from build123d import *

# Parameters (mm, degrees)
SKETCH_1_R                        = 1.6
SM_BASE_FLANGE_1_DEPTH            = 1
SKETCH_2_R                        = 3
EXTRUDE_1_DEPTH                   = 2
HOLE_WIZARD_M3_1_D                = 2.5
SM_EDGE_FLANGE_1_STRIP_W          = 6
SM_EDGE_FLANGE_1_STRIP_H          = 1
SM_EDGE_FLANGE_1_STRIP_CUT_DEPTH  = 177.34
SM_EDGE_FLANGE_1_RELIEF_W         = 8
SM_EDGE_FLANGE_1_RELIEF_H         = 2
SM_EDGE_FLANGE_1_RELIEF_CUT_DEPTH = 1
SM_EDGE_FLANGE_1_DEPTH            = 177.34
SM_EDGE_FLANGE_1_FLAT_DEPTH       = 1
SKETCH_8_R                        = 3
EXTRUDE_2_DEPTH                   = 2
HOLE_WIZARD_M3_2_D                = 2.5


# Sheet-metal steps are written as plain solids
with BuildPart() as part:
    # Sketch 1 → 基体-法兰1 (new body)
    with BuildSketch(Plane(origin=(0, 0, 0), x_dir=(1, 0, 0), z_dir=(0, 1, 0))):
        with BuildLine():
            Line((-113.67, 31.388001247), (-113.67, -28.611998753))
            ThreePointArc((-113.67, -28.611998753), (-112.791320344, -30.733319096), (-110.67, -31.611998753))
            Line((-110.67, -31.611998753), (110.67, -31.611998753))
            ThreePointArc((110.67, -31.611998753), (112.791320344, -30.733319096), (113.67, -28.611998753))
            Line((113.67, -28.611998753), (113.67, -8.25463944))
            ThreePointArc((113.67, -8.25463944), (113.441638598, -7.106589143), (112.791320344, -6.133319096))
            Line((112.791320344, -6.133319096), (55.148679656, 51.509321591))
            ThreePointArc((55.148679656, 51.509321591), (54.17540961, 52.159639845), (53.027359313, 52.388001247))
            Line((53.027359313, 52.388001247), (-2.67, 52.388001247))
            ThreePointArc((-2.67, 52.388001247), (-4.084213562, 51.80221481), (-4.67, 50.388001247))
            Line((-4.67, 50.388001247), (-4.67, 33.388001247))
            Line((-4.67, 33.388001247), (-111.67, 33.388001247))
            ThreePointArc((-111.67, 33.388001247), (-113.084213562, 32.80221481), (-113.67, 31.388001247))
        make_face()
        with Locations(Location((-105.67, -13.611998753, 0), (0, 0, 270))):
            Circle(SKETCH_1_R, mode=Mode.SUBTRACT)
        with Locations(Location((-105.67, 13.388001247, 0), (0, 0, 270))):
            Circle(SKETCH_1_R, mode=Mode.SUBTRACT)
        with Locations(Location((-89.67, 25.388001247, 0), (0, 0, 270))):
            Circle(SKETCH_1_R, mode=Mode.SUBTRACT)
        with Locations(Location((-25.67, 25.388001247, 0), (0, 0, 270))):
            Circle(SKETCH_1_R, mode=Mode.SUBTRACT)
        with Locations(Location((22.33, 44.388001247, 0), (0, 0, 270))):
            Circle(SKETCH_1_R, mode=Mode.SUBTRACT)
        with Locations(Location((60.516291501, 34.828001247, 0), (0, 0, 270))):
            Circle(SKETCH_1_R, mode=Mode.SUBTRACT)
        with Locations(Location((96.116291501, -0.771998753, 0), (0, 0, 270))):
            Circle(SKETCH_1_R, mode=Mode.SUBTRACT)
        with Locations(Location((105.67, -19.111998753, 0), (0, 0, 270))):
            Circle(SKETCH_1_R, mode=Mode.SUBTRACT)
        with BuildLine():
            Line((-43.83, 11.388001247), (5.17, 11.388001247))
            ThreePointArc((5.17, 11.388001247), (5.523553391, 11.241554638), (5.67, 10.888001247))
            Line((5.67, 10.888001247), (5.67, -16.111998753))
            ThreePointArc((5.67, -16.111998753), (5.523553391, -16.465552143), (5.17, -16.611998753))
            Line((5.17, -16.611998753), (-43.83, -16.611998753))
            ThreePointArc((-43.83, -16.611998753), (-44.183553391, -16.465552143), (-44.33, -16.111998753))
            Line((-44.33, -16.111998753), (-44.33, 10.888001247))
            ThreePointArc((-44.33, 10.888001247), (-44.183553391, 11.241554638), (-43.83, 11.388001247))
        make_face(mode=Mode.SUBTRACT)
    extrude(amount=-SM_BASE_FLANGE_1_DEPTH)

    # Sketch 2 → 凸台-拉伸1 (add)
    with BuildSketch(Plane.XZ.offset(1)):
        with Locations(Location((-19.33, -17.388001247, 0), (0, 0, 90))):
            Circle(SKETCH_2_R)
        with Locations(Location((-19.33, 22.611998753, 0), (0, 0, 90))):
            Circle(SKETCH_2_R)
    extrude(amount=EXTRUDE_1_DEPTH)

    # M3 螺纹孔1 (through all)
    with Locations(Plane(origin=(0, -3, 0), x_dir=(-1, 0, 0), z_dir=(0, -1, 0))):
        with Locations((19.33, 17.388001247), (19.33, -22.611998753)):
            Hole(HOLE_WIZARD_M3_1_D / 2)

    # 边线-法兰1 strip (across the edge) → 边线-法兰1 strip cut (cut)
    with BuildSketch(Plane(origin=(88.67, -1, 31.611998753), x_dir=(0, 0, -1), z_dir=(-1, 0, 0))):
        with Locations((-1, -0.5)):
            Rectangle(SM_EDGE_FLANGE_1_STRIP_W, SM_EDGE_FLANGE_1_STRIP_H)
    extrude(amount=SM_EDGE_FLANGE_1_STRIP_CUT_DEPTH, mode=Mode.SUBTRACT)

    # 边线-法兰1 relief (on the sheet) → 边线-法兰1 relief cut (cut)
    with BuildSketch(Plane(origin=(88.67, -1, 29.611998753), x_dir=(0, 0, -1), z_dir=(0, -1, 0))):
        with Locations((-2, 1)):
            Rectangle(SM_EDGE_FLANGE_1_RELIEF_W, SM_EDGE_FLANGE_1_RELIEF_H)
        with Locations((-2, -178.34)):
            Rectangle(SM_EDGE_FLANGE_1_RELIEF_W, SM_EDGE_FLANGE_1_RELIEF_H)
    extrude(amount=-SM_EDGE_FLANGE_1_RELIEF_CUT_DEPTH, mode=Mode.SUBTRACT)

    # 边线-法兰1 bend section (across the edge) → 边线-法兰1 (add)
    with BuildSketch(Plane(origin=(88.67, -1, 31.611998753), x_dir=(0, 0, -1), z_dir=(-1, 0, 0))):
        with BuildLine():
            Line((0, 1), (1, 1))
            ThreePointArc((1, 1), (1.292893219, 0.292893219), (2, 0))
            Line((2, 0), (2, -1))
            ThreePointArc((2, -1), (0.585786438, -0.414213562), (0, 1))
        make_face()
    extrude(amount=SM_EDGE_FLANGE_1_DEPTH)

    # 边线-法兰1 profile (on flange) → 边线-法兰1 flat (add)
    with BuildSketch(Plane(origin=(0, -1, 31.611998753), x_dir=(-1, 0, 0), z_dir=(0, 0, 1))):
        with BuildLine():
            Line((83.67, 12.5), (-83.67, 12.5))
            ThreePointArc((-83.67, 12.5), (-87.205533906, 11.035533906), (-88.67, 7.5))
            Line((-88.67, 7.5), (-88.67, 1))
            Line((-88.67, 1), (88.67, 1))
            Line((88.67, 1), (88.67, 7.5))
            ThreePointArc((88.67, 7.5), (87.205533906, 11.035533906), (83.67, 12.5))
        make_face()
    extrude(amount=-SM_EDGE_FLANGE_1_FLAT_DEPTH)

    # 草图8 → 凸台-拉伸2 (add)
    with BuildSketch(Plane(origin=(0, 0, 30.611998753), x_dir=(-1, 0, 0), z_dir=(0, 0, -1))):
        with Locations(Location((-0.17, -8.5, 0), (0, 0, 270))):
            Circle(SKETCH_8_R)
    extrude(amount=EXTRUDE_2_DEPTH)

    # M3 螺纹孔2 (through all)
    with Locations(Plane(origin=(0, 0, 28.611998753), x_dir=(-1, 0, 0), z_dir=(0, 0, -1))):
        with Locations((-0.17, -8.5)):
            Hole(HOLE_WIZARD_M3_2_D / 2)


solid = part.part
Verification items for the finished model (mm, model axes). A direction names the side the tool comes from. Round coordinates to 2 decimals unless told otherwise and drop trailing zeros. Order: outer loops, then holes, each group sorted by start corner. A loop starts at its lowest first (then second) coordinate and runs counter-clockwise, first axis right, second up.
1. Section check A-A on x = -31. Record the cut outline in (y, z), then the cut area to 3 significant figures.
Final values:
outline: (-13.5, 30.61) - (-2, 30.61) arc R1 cw to (-1, 29.61) - (-1, 16.61) - (0, 16.61) - (0, 29.61) arc R2 ccw to (-2, 31.61) - (-13.5, 31.61) - close; (-1, -33.39) - (0, -33.39) - (0, -11.39) - (-1, -11.39) - close
area: 48.9 mm2
2. Go/stop test with flat-tipped pins: P1, Ø1.8, axis at x = -0.5, y = -9.5, coming from the -Z side; P2, Ø1.1, axis at x = 90, y = -0.5, coming from the +Z side; P3, Ø2, axis at x = 50, y = -3.5, coming from the -Z side. Record where each tip stops, or that it passes through.
Final values:
P1: stops at z = 28.61
P2: stops at z = 27.61
P3: stops at z = 30.61
3. Access from +Z, -Z, +X, -X, +Y, -Y to the whole of each face (thin tool, end or side, straight path). Record for faces 1 (the flat face through (-19, -3, 24)), 2 (the cylindrical face through (-20.231, -1.986, -14.527)), 3 (the cylindrical face through (1.32, -11.27, 29.63)), 4 (the flat face through (88.67, -4, 31)).
Final values:
face 1: -Z, +X, -X, -Y
face 2: -Y
face 3: -Z
face 4: +Z, +Y, -Y
4. Release check for a two-part mould opening along Z. For faces 5 (the flat face through (1, -7, 31.612)), 6 (the cylindrical face through (-21.86, -1.986, 24.225)), 7 (the flat face through (-88.67, -3, 31)), 8 (the flat face through (0, -10, 28.612)) record: +Z half, -Z half, draft (parallel to the pull), parting line (faces both ways), or undercut.
Final values:
face 5: +Z half
face 6: undercut
face 7: draft
face 8: -Z half
5. Thickness scan on L1, parallel to Z at x = -105.67, y = -0.2; L2, parallel to Z at x = 105.67, y = -0.35; L3, parallel to Z at x = -19.33, y = -1.1. Record the ranges inside material, lowest first.
Final values:
L1: z = -33.39 to -14.99, -11.79 to 12.01, 15.21 to 31.61
L2: z = -0.99 to 17.51, 20.71 to 31.61
L3: z = -20.39 to -18.64, -16.14 to -14.39, 19.61 to 21.36, 23.86 to 25.61, 30.05 to 31.4
